Geometry: final body of the model. Coordinates: model frame, mm. A direction names the side the tool comes from. Coordinates: 2 decimals unless noted, no trailing zeros. Order: outer loops, then holes, each group sorted by start corner. A loop starts at its lowest first (then second) coordinate and runs counter-clockwise, first axis right, second up. Notation, with made-up numbers: M 28,0.5 L 60,0.5 A7 cw 60,13.5 Z; hole C -19,39.25 d7. An arc over 180 degrees is marked long. Write item = value, one per line.
from build123d import *

# Parameters (mm, degrees)
SKETCH_2_R               = 2
CUT_EXTRUDE_1_DEPTH      = 42.761704946
PATTERN_CIRCULAR_1_COUNT = 2
PATTERN_CIRCULAR_1_ANGLE = 120
CHAMFER_1_SIZE           = 0.675


with BuildPart() as part:
    # Эскиз1 → Повернуть1 (revolve)
    with BuildSketch(Plane.XY, mode=Mode.PRIVATE) as revolve_1_sk:
        with BuildLine():
            Line((-8.5, 24.571324751), (-8.5, 15.875))
            Line((-8.5, 15.875), (-14.3, 15.875))
            Line((-14.3, 15.875), (-14.3, 12.5))
            Line((-14.3, 12.5), (19.8, 12.5))
            Line((19.8, 12.5), (19.8, 15.875))
            Line((19.8, 15.875), (8.5, 15.875))
            Line((8.5, 15.875), (8.5, 24.571324751))
            ThreePointArc((8.5, 24.571324751), (0, 26), (-8.5, 24.571324751))
        make_face()
    revolve(revolve_1_sk.sketch.rotate(Axis((-1000, 0, 0), (1, 0, 0)), 90), axis=Axis((-1000, 0, 0), (1, 0, 0)))

    # Эскиз2 → Вырез-Вытянуть1 (cut, through all)
    with BuildSketch(Plane(origin=(0, 0, 0), x_dir=(1, 0, 0), z_dir=(0, 1, 0))):
        with Locations(Location((14.15, 0, 0), (0, 0, 90))):
            Circle(SKETCH_2_R)
    cut_extrude_1 = extrude(amount=CUT_EXTRUDE_1_DEPTH, mode=Mode.SUBTRACT)

    # Круговой массив1: Вырез-Вытянуть1 ×2 about axis
    pattern_circular_1_axis = Axis((-1000, 0, 0), (-1, 0, 0))
    for i in range(1, PATTERN_CIRCULAR_1_COUNT):
        add(cut_extrude_1.rotate(pattern_circular_1_axis, i * PATTERN_CIRCULAR_1_ANGLE / (PATTERN_CIRCULAR_1_COUNT - 1)), mode=Mode.SUBTRACT)

    # Фаска1
    chamfer_1_edges = [part.edges().sort_by_distance(p)[0] for p in [
        (-14.3, 0, -15.875),
        (-14.3, 0, -12.5),
        (19.8, 0, -12.5),
        (19.8, 0, -15.875),
    ]]
    chamfer(chamfer_1_edges, length=CHAMFER_1_SIZE)


solid = part.part
1) Section B-B, the plane x = 14.15. Return loops of the section in (y, z) (3 decimals).
Numbers:
outline = M -9.606,-12.639 L -7.902,-9.686 A12.5 cw long 12.339,2 L 15.749,2 A15.875 ccw long Z; M -6.142,-14.639 A15.875 ccw 15.749,-2 L 12.339,-2 A12.5 cw -4.437,-11.686 Z
2) Section C-C, the plane y = 0. Return loops of the section in (x, z) (3 decimals), and give its area (3 significant figures).
Numbers:
outline = M -14.3,-15.2 L -13.625,-15.875 L -8.5,-15.875 L -8.5,-24.571 A26 ccw 8.5,-24.571 L 8.5,-15.875 L 19.125,-15.875 L 19.8,-15.2 L 19.8,-13.175 L 19.125,-12.5 L -13.625,-12.5 L -14.3,-13.175 Z; M -14.3,13.175 L -13.625,12.5 L 19.125,12.5 L 19.8,13.175 L 19.8,15.2 L 19.125,15.875 L 8.5,15.875 L 8.5,24.571 A26 ccw -8.5,24.571 L -8.5,15.875 L -13.625,15.875 L -14.3,15.2 Z
area = 557 mm²
3) Line query: L1, parallel to Y at x = 9, z = 0 (3 decimals); L2, parallel to X at y = 17, z = 2; L3, parallel to Z at x = 14.15, y = 14.5. Output: solid intervals per line, ascending.
Numbers:
L1 = -15.875 to -12.5, 12.5 to 15.875
L2 = -8.5 to 8.5
L3 = -6.46 to -2, 2 to 6.46
4) Pin query (flat end, axial travel): pin 1 (4.5 mm diameter, centred on x = 14.15, z = 0, fed in from -Y) (3 decimals); pin 2 (6 mm diameter, centred on x = 8.5, y = 3.5, fed in from -Z); pin 3 (6 mm diameter, centred on x = -8, z = 3.5, fed in from +Y). Return the tip coordinate at first contact, or that it passes through.
Numbers:
pin_1 = -15.875
pin_2 = -25.25
pin_3 = 25.36
5) Section A-A, the plane z = 0. Return loops of the section in (x, y) (3 decimals), and give its area (3 significant figures).
Numbers:
outline = M -14.3,-15.2 L -13.625,-15.875 L -8.5,-15.875 L -8.5,-24.571 A26 ccw 8.5,-24.571 L 8.5,-15.875 L 19.125,-15.875 L 19.8,-15.2 L 19.8,-13.175 L 19.125,-12.5 L -13.625,-12.5 L -14.3,-13.175 Z; M -14.3,13.175 L -13.625,12.5 L 12.15,12.5 L 12.15,15.875 L 8.5,15.875 L 8.5,24.571 A26 ccw -8.5,24.571 L -8.5,15.875 L -13.625,15.875 L -14.3,15.2 Z; M 16.15,12.5 L 19.125,12.5 L 19.8,13.175 L 19.8,15.2 L 19.125,15.875 L 16.15,15.875 Z
area = 543 mm²
6) Section D-D, the plane x = 10. Return loops of the section in (y, z) (3 decimals).
Numbers:
outline = C 0,0 d31.75; hole C 0,0 d25
7) Mould query, pull axis Y, two halves, no side actions, for faces 1 (the face through (-11.098, 15.497, -3.441)), 2 (the face through (19.8, -14, 0)), 3 (the face through (15.4, -5.7, -13)). Classes: pulls with the +Y half, pulls with the -Y half, needs draft (parallel to the pull), parting line crosses it, or undercut.
Numbers:
face_1 = parting line crosses it
face_2 = needs draft
face_3 = undercut
8) Set-up query: faces 4 (the face through (14.1, 14.1, 2)), 5 (the face through (8.5, 16.04, 0.34)), 6 (the face through (-14.3, -14, 0)), 7 (the face through (-8.5, 16.04, -0.34)). Return all of +Z, -Z, +X, -X, +Y, -Y with unobstructed straight access to the full face (end or side cutting, diameter ignored); none if empty.
Numbers:
face_4 = +Y
face_5 = +X
face_6 = +Z, -Z, -X, +Y, -Y
face_7 = -X
